CAD build for the part. Positions are in the model's coordinates, mm. Coordinates: 2 decimals unless noted, no trailing zeros. Loops run counter-clockwise (first coordinate to the right, second up) from the corner with the lowest first, then second, coordinate; pieces in that order, holes last. Notation, with made-up numbers: (-14.75, -7.75) - (4.25, -7.75) arc R16 ccw to (4.25, 5.25) - close; hole circle Ø3 at (31, -30.5). An arc over 180 degrees is marked (long way). Put each result on its own line as item: value.
```python
from build123d import *

# Parameters (mm, degrees)
SKETCH1_W           = 192
SKETCH1_H           = 55
BOSS_EXTRUDE1_DEPTH = 8
SKETCH2_R           = 4
SKETCH2_R_2         = 1.6
CUT_EXTRUDE2_DEPTH  = 9


with BuildPart() as part:
    # Sketch1 → Boss-Extrude1 (new body)
    with BuildSketch(Plane.XY):
        Rectangle(SKETCH1_W, SKETCH1_H)
    extrude(amount=BOSS_EXTRUDE1_DEPTH)

    # Sketch2 → Cut-Extrude2 (cut)
    with BuildSketch(Plane.XY):
        with Locations(Location((0, 0, 0), (0, 0, 180))):
            Circle(SKETCH2_R)
        with Locations(Location((-90, 12, 0), (0, 0, 180))):
            Circle(SKETCH2_R_2)
        with Locations(Location((-90, -12, 0), (0, 0, 180))):
            Circle(SKETCH2_R_2)
        with Locations(Location((90, 12, 0), (0, 0, 180))):
            Circle(SKETCH2_R_2)
        with Locations(Location((90, -12, 0), (0, 0, 180))):
            Circle(SKETCH2_R_2)
    extrude(amount=CUT_EXTRUDE2_DEPTH, mode=Mode.SUBTRACT)


solid = part.part
```
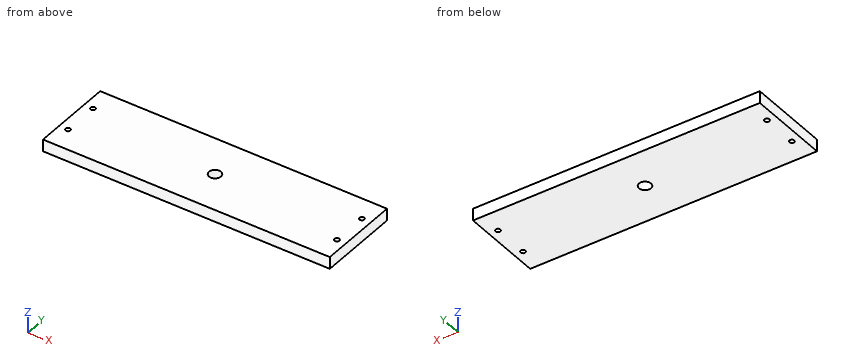
Q1. Slice it at B-B, the plane y = -12. Give the cut face in (x, z), then the cut area to 3 significant figures.
Determined:
outline: (-96, 0) - (-91.6, 0) - (-91.6, 8) - (-96, 8) - close; (-88.4, 0) - (88.4, 0) - (88.4, 8) - (-88.4, 8) - close; (91.6, 0) - (96, 0) - (96, 8) - (91.6, 8) - close
area: 1,480 mm2
Q2. Slice it at C-C, the plane x = 0. Give the cut face in (y, z), then the cut area to 3 significant figures.
Determined:
outline: (-27.5, 0) - (-4, 0) - (-4, 8) - (-27.5, 8) - close; (4, 0) - (27.5, 0) - (27.5, 8) - (4, 8) - close
area: 376 mm2
Q3. Wall check: L1, parallel to X at y = 12, z = 2.25; L2, parallel to Y at x = -90, z = 6.5. Give the ranges that are in metal, low to high. Write a range as from..to.
Determined:
L1: -96..-91.6, -88.4..88.4, 91.6..96
L2: -27.5..-13.6, -10.4..10.4, 13.6..27.5
Q4. Slice it at D-D, the plane y = 0. Give the cut face in (x, z).
Determined:
outline: (-96, 0) - (-4, 0) - (-4, 8) - (-96, 8) - close; (4, 0) - (96, 0) - (96, 8) - (4, 8) - close
Q5. Slice it at A-A, the plane x = -90. Give the cut face in (y, z), then the cut area to 3 significant figures.
Determined:
outline: (-27.5, 0) - (-13.6, 0) - (-13.6, 8) - (-27.5, 8) - close; (-10.4, 0) - (10.4, 0) - (10.4, 8) - (-10.4, 8) - close; (13.6, 0) - (27.5, 0) - (27.5, 8) - (13.6, 8) - close
area: 389 mm2
